```python
from build123d import *

# Parameters (mm, degrees)
CUT_EXTRUDE_START   = 10
CUT_EXTRUDE_2_DEPTH = 144.502052104
CHAMFER_1_SIZE      = 2
CHAMFER_2_SIZE      = 2


with BuildPart() as part:
    # Эскиз1 → Повернуть1 (revolve)
    with BuildSketch(Plane.XY, mode=Mode.PRIVATE) as revolve_1_sk:
        Polygon((0, 0), (0, -12.5), (26, -12.5), (26, -15), (62, -15), (62, -18), (70, -18), (70, -28.8), (120, -28.8), (120, -15), (134, -15), (134, -12.5), (148, -12.5), (148, 0), align=None)
    revolve(revolve_1_sk.sketch.rotate(Axis((148, 0, 0), (-1, 0, 0)), 180), axis=Axis((148, 0, 0), (-1, 0, 0)))

    # Эскиз3 → Вырез-Повернуть1 (revolve, cut)
    with BuildSketch(Plane.XY, mode=Mode.PRIVATE) as cut_revolve_1_sk:
        Polygon((0, 0), (10.054700538, 0), (8.9, 2), (3.9, 2), (0, 4.25), align=None)
    cut_revolve_1 = revolve(cut_revolve_1_sk.sketch.rotate(Axis((0, 0, 0), (1, 0, 0)), 90), axis=Axis((0, 0, 0), (1, 0, 0)), mode=Mode.SUBTRACT)

    # Зеркальное отражение1: Вырез-Повернуть1 across plane
    add(cut_revolve_1.mirror(Plane.ZY.offset(-74)), mode=Mode.SUBTRACT)

    # Эскиз4 → Вырез-Вытянуть2 (cut, through all)
    with BuildSketch(Plane.XY.offset(CUT_EXTRUDE_START)):
        with BuildLine():
            Line((33, 4), (55, 4))
            ThreePointArc((55, 4), (59, 0), (55, -4))
            Line((55, -4), (33, -4))
            ThreePointArc((33, -4), (29, 0), (33, 4))
        make_face()
    extrude(amount=CUT_EXTRUDE_2_DEPTH, mode=Mode.SUBTRACT)

    # Фаска1
    chamfer_1_edges = [part.edges().sort_by_distance(p)[0] for p in [
        (0, -12.5, 0),
    ]]
    chamfer(chamfer_1_edges, length=CHAMFER_1_SIZE)

    # Фаска2
    chamfer_2_edges = [part.edges().sort_by_distance(p)[0] for p in [
        (148, -12.5, 0),
        (120, -28.8, 0),
        (70, -28.8, 0),
    ]]
    chamfer(chamfer_2_edges, length=CHAMFER_2_SIZE)


solid = part.part
```
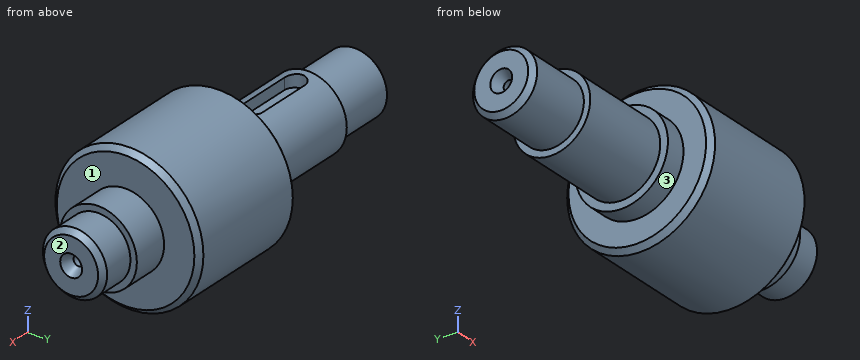
Can you work these out from the model? Positions are in its coordinate system, mm. Face numbers are marked on the shaded views. A direction names the side the tool comes from. Coordinates: 2 decimals unless noted, no trailing zeros. Loops run counter-clockwise (first coordinate to the right, second up) from the corner with the lowest first, then second, coordinate; pieces in that order, holes last.
Item 1: Which directions (+Z, -Z, +X, -X, +Y, -Y) give clear straight access to the entire face, cutting with the end or side of a thin tool? Please do the marked faces 1, 2 and 3.
Answers below:
face 1: +X
face 2: +Z, -Z, +X, +Y, -Y
face 3: -X
Item 2: Suppose I cut it at B-B (x = 91). Please give me the cut outline in (y, z), then the cut area to 3 significant figures.
Answers below:
outline: circle Ø57.6 at (0, 0)
area: 2,610 mm2
Item 3: Suppose I cut it at C-C (x = 36.5). Please give me the cut outline in (y, z).
Answers below:
outline: (-4, 10) - (-4, 14.46) arc R15 ccw (long way) to (4, 14.46) - (4, 10) - close
Item 4: Suppose I cut it at A-A (x = 130). Please give me the cut outline in (y, z).
Answers below:
outline: circle Ø30 at (0, 0)
Item 5: I'm going to push flat-ended pins straight in: pin 1 (1.3 mm diameter, centred on x = 49, z = 12.5, fed in from -Y); pin 2 (3 mm diameter, centred on x = 30, y = -9, fed in from +Z); pin 3 (4 mm diameter, centred on y = -21, z = 0.5, fed in from -X). Where does each tip first touch, or does it pass through?
Answers below:
pin 1: stops at y = -9.2
pin 2: stops at z = 12.99
pin 3: stops at x = 70
Item 6: Please list where these lines run through material, in increasing order: L1, parallel to X at y = -22.5, z = 1.5; L2, parallel to X at y = 21, z = 18.5; L3, parallel to Z at x = 114, y = -18.5.
Answers below:
L1: x = 70 to 120
L2: x = 71.19 to 118.81
L3: z = -22.07 to 22.07
